Input: dimensioned drawing with shaded views. Units: mm. Origin: part minimum x, y, z. A direction names the side the tool comes from. Give positions to 0.01 mm unless a question says otherwise; leave off trailing zeros. Write each loop counter-clockwise with the first axis right and the second up, starting at its lowest first coordinate (ties: lowest second). Pieces come first, ordered by that corner, then holes. Notation, with made-up numbers: M 64.5,14.25 L 114.5,14.25 A34 ccw 114.5,52.25 Z; hole C 82,-28.75 d1. An arc over 180 degrees is marked long. Answer as a JSON object with one key per item and string values.
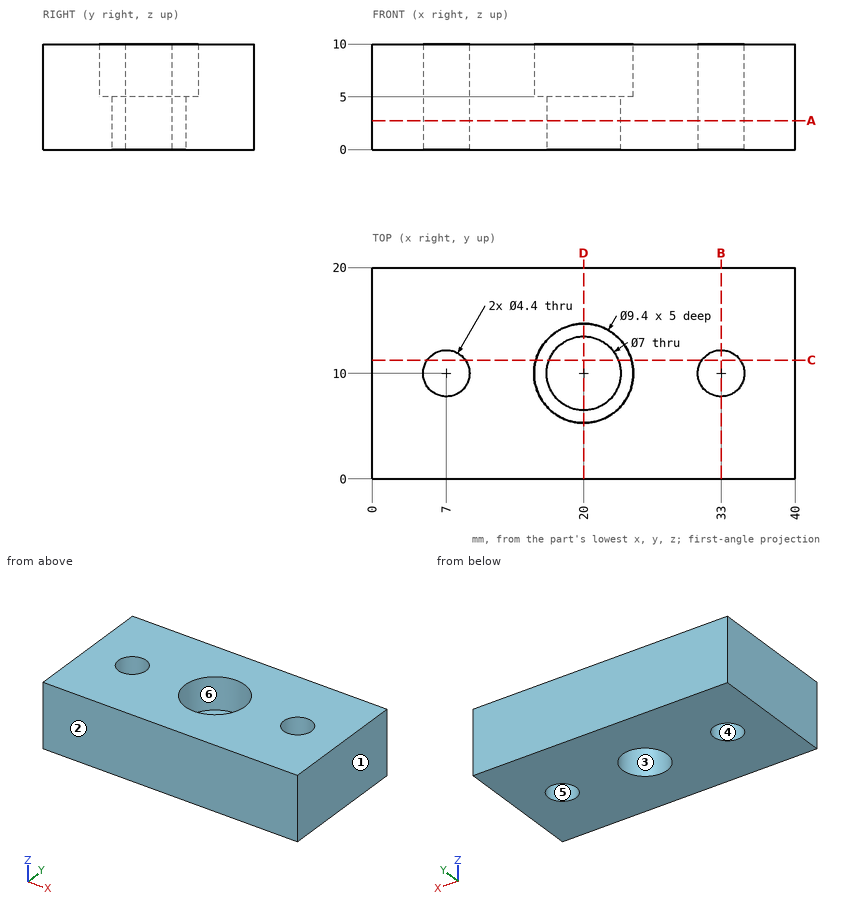
1) Line query: line 1 (X direction, y = 10, z = 4.5); line 2 (X direction, y = 10, z = 6.3); line 3 (Y direction, x = 20, z = 3.25). Output: solid intervals per line, ascending. Write a range as from..to.
Geometry check:
{"line 1": "x = 0..4.8, 9.2..16.5, 23.5..30.8, 35.2..40", "line 2": "x = 0..4.8, 9.2..15.3, 24.7..30.8, 35.2..40", "line 3": "y = 0..6.5, 13.5..20"}
2) Cut plane C-C on y = 11.25. Return loops of the section in (x, z), and give its area (3 significant figures).
Geometry check:
{"outline": "M 0,0 L 5.19,0 L 5.19,10 L 0,10 Z; M 8.81,0 L 16.73,0 L 16.73,5 L 15.47,5 L 15.47,10 L 8.81,10 Z; M 23.27,0 L 31.19,0 L 31.19,10 L 24.53,10 L 24.53,5 L 23.27,5 Z; M 34.81,0 L 40,0 L 40,10 L 34.81,10 Z", "area": "250 mm2"}
3) Cut plane B-B on x = 33. Return loops of the section in (y, z).
Geometry check:
{"outline": "M 0,0 L 7.8,0 L 7.8,10 L 0,10 Z; M 12.2,0 L 20,0 L 20,10 L 12.2,10 Z"}
4) Set-up query: the marked faces 5 and 6. Return all of +Z, -Z, +X, -X, +Y, -Y with unobstructed straight access to the full face (end or side cutting, diameter ignored); none if empty.
Geometry check:
{"face 5": "+Z, -Z", "face 6": "+Z"}
5) Contact query for a flat-ended pin moving along its axis: P1, Ø3, axis at x = 20, y = 9, coming from the +Z side. Output: stop coordinate, or through.
Geometry check:
{"P1": "passes through"}
6) Cut plane A-A on z = 2.75. Return loops of the section in (x, y).
Geometry check:
{"outline": "M 0,0 L 40,0 L 40,20 L 0,20 Z; hole C 7,10 d4.4; hole C 20,10 d7; hole C 33,10 d4.4"}
7) Cut plane D-D on x = 20. Return loops of the section in (y, z).
Geometry check:
{"outline": "M 0,0 L 6.5,0 L 6.5,5 L 5.3,5 L 5.3,10 L 0,10 Z; M 13.5,0 L 20,0 L 20,10 L 14.7,10 L 14.7,5 L 13.5,5 Z"}
8) Pull-direction query (Y, two-part tool) for the marked faces 1, 2, 3 and 4; classes: pulls with the +Y half, pulls with the -Y half, needs draft (parallel to the pull), parting line crosses it, or undercut.
Geometry check:
{"face 1": "needs draft", "face 2": "pulls with the -Y half", "face 3": "undercut", "face 4": "undercut"}
